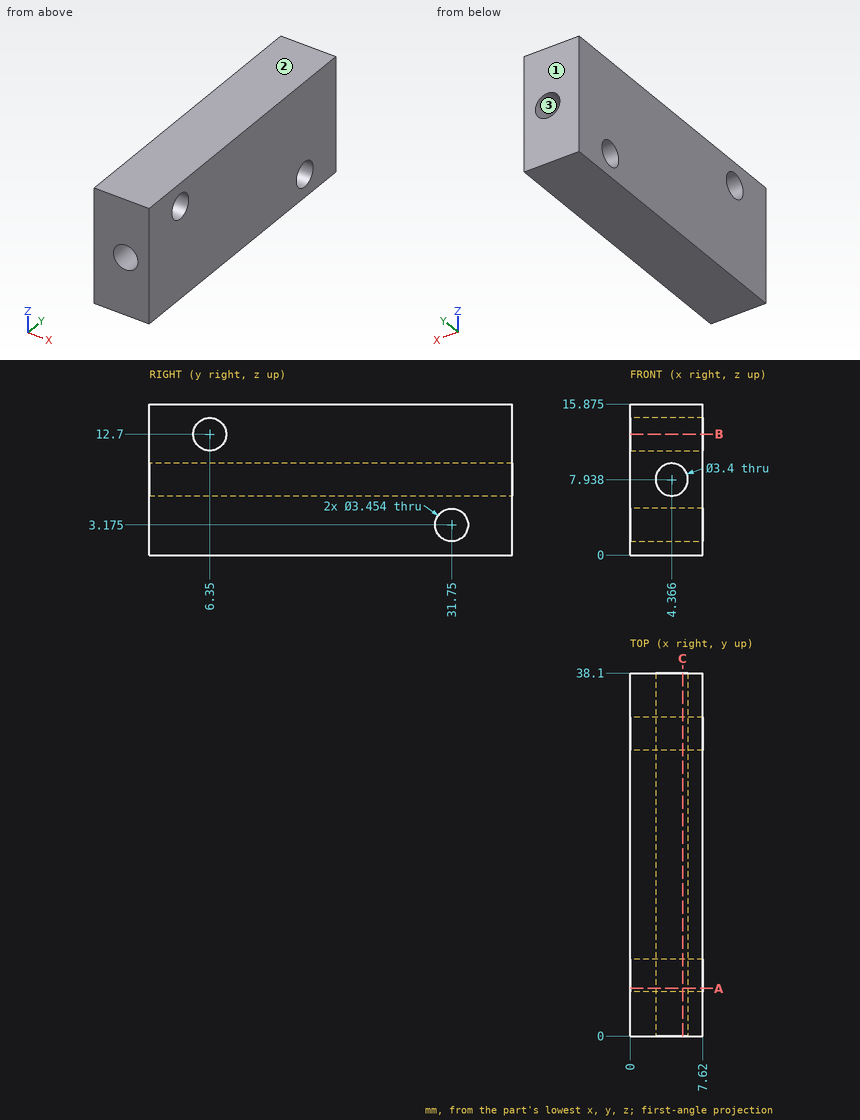
Answer from the drawing. Dimensions are ordinates in mm from the lowest x, y and z of the part. Coordinates: 2 decimals unless noted, no trailing zeros. Write each loop counter-clockwise with the first axis right and the second up, starting at its lowest first coordinate (ties: lowest second). Pieces come first, ordered by that corner, then holes. Notation, with made-up numbers: (-35, -30.5) -> (-6, -30.5) arc R21 ccw to (-6, -25.5) -> close; hole circle Ø9 at (62, -22). An arc over 180 degrees is marked (long way). One line per question, with ' | ' between items.
1. Straight lines are drawn through the part: line 1 (Y direction, x = 4.75, z = 12.7); line 2 (Z direction, x = 4.25, y = 23) (1 decimal); line 3 (Y direction, x = 3.5, z = 4.5) (1 decimal). For each, find the intervals that lie inside material, in ascending order.
Verdict:
line 1: y = 0 to 4.62, 8.08 to 38.1 | line 2: z = 0 to 6.2, 9.6 to 15.9 | line 3: y = 0 to 30.6, 32.9 to 38.1
2. Section B-B (z = 12.7) is taken. Determine the outline of the cut face in (x, y).
Verdict:
outline: (0, 0) -> (7.62, 0) -> (7.62, 4.62) -> (0, 4.62) -> close; (0, 8.08) -> (7.62, 8.08) -> (7.62, 38.1) -> (0, 38.1) -> close
3. Section A-A (y = 5) is taken. Determine the outline of the cut face in (x, z) (1 decimal).
Verdict:
outline: (0, 0) -> (7.6, 0) -> (7.6, 11.6) -> (0, 11.6) -> close; (0, 13.8) -> (7.6, 13.8) -> (7.6, 15.9) -> (0, 15.9) -> close; hole circle Ø3.4 at (4.4, 7.9)
4. Section C-C (x = 5.5) is taken. State how many separate pieces and enclosed holes the cut face has.
Verdict:
separate pieces: 2 | enclosed holes: 2
5. For a pull along Z with two mould halves and no side action, classify the marked faces 1, 2 and 3 as released by +Z, released by -Z, zero draft, split by the parting line, or undercut.
Verdict:
face 1: zero draft | face 2: released by +Z | face 3: undercut
6. Given pin 1 Ø3 at (y, z) = (31.75, 3.175) entering from -X, flat-ended and moving along its own axis, determine where the tip first touches the part or whether it passes through.
Verdict:
pin 1: passes through
